```python
from build123d import *

# Parameters (mm, degrees)
SKETCH1_R               = 16.7005
SKETCH1_R_2             = 13.335
BOSS_EXTRUDE1_DEPTH     = 520.7
SKETCH3_R               = 16.7005
SKETCH3_R_2             = 13.335
BOSS_EXTRUDE2_DEPTH     = 660.4
SKETCH2_R               = 6.35
CUT_EXTRUDE1_DEPTH      = 17.7005
CUT_EXTRUDE1_DEPTH_BACK = 17.7005


with BuildPart() as part:
    # Sketch1 → Boss-Extrude1 (new body)
    with BuildSketch(Plane(origin=(0, 0, 0), x_dir=(1, 0, 0), z_dir=(0, 1, 0))):
        Circle(SKETCH1_R)
        Circle(SKETCH1_R_2, mode=Mode.SUBTRACT)
    extrude(amount=BOSS_EXTRUDE1_DEPTH)

    # Sketch3 → Boss-Extrude2 (add)
    with BuildSketch(Plane.XZ):
        Circle(SKETCH3_R)
        Circle(SKETCH3_R_2, mode=Mode.SUBTRACT)
    extrude(amount=BOSS_EXTRUDE2_DEPTH)

    # Sketch2 → Cut-Extrude1 (cut, two sides)
    with BuildSketch(Plane(origin=(0, 0, 0), x_dir=(0, 0, -1), z_dir=(1, 0, 0))) as cut_extrude1_sk:
        with Locations((0, -69.85)):
            Circle(SKETCH2_R)
    extrude(amount=CUT_EXTRUDE1_DEPTH, mode=Mode.SUBTRACT)
    extrude(cut_extrude1_sk.sketch, amount=-CUT_EXTRUDE1_DEPTH_BACK, mode=Mode.SUBTRACT)


solid = part.part
```
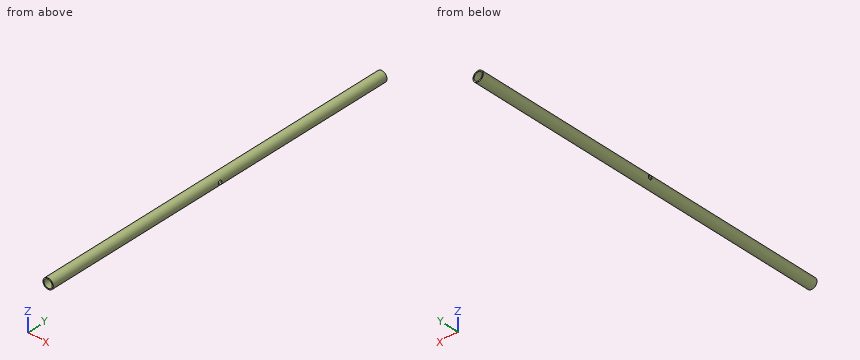
Part model, mm, in its own coordinate system. Coordinates: 2 decimals unless noted, no trailing zeros. Order: outer loops, then holes, each group sorted by start corner. A loop starts at its lowest first (then second) coordinate and runs counter-clockwise, first axis right, second up. Notation, with made-up numbers: (-6.5, -39) -> (50.5, -39) arc R16 cw to (50.5, -29) -> close; hole circle Ø9 at (-19, 31.5). An arc over 180 degrees is marked (long way). Put each result on its own line as item: value. Start each with the question number.
(1) Pin check, flat tips, straight feed: pin 1 Ø1 at (y, z) = (-254, 9) entering from +X; pin 2 Ø2 at (x, y) = (-7.5, 79) entering from +Z; pin 3 Ø4 at (x, y) = (3.5, -176.5) entering from +Z. Stop position of each tip, or through.
(2) Probe line 1 along X through (y, z) = (134.5, 1); line 2 along Z through (x, y) = (0, -124) (1 decimal); line 3 along X through (y, z) = (-53, -2). List the from-to ranges inside material, lowest first. Write a range as [from, to].
(3) Band-saw the part on C-C (y = 378). Give the cut face in (x, z) (1 decimal).
(4) Band-saw the part on A-A (x = 0). Give the cut face in (y, z) (1 decimal), then the cut area to 3 significant figures.
(5) Band-saw the part on B-B (z = 0). Give the cut face in (x, y) (1 decimal), then the cut area to 3 significant figures.
Determined:
1. pin 1: stops at x = 14.38
1. pin 2: stops at z = 15.38
1. pin 3: stops at z = 16.63
2. line 1: x = [-16.67, -13.3], [13.3, 16.67]
2. line 2: z = [-16.7, -13.3], [13.3, 16.7]
2. line 3: x = [-16.58, -13.18], [13.18, 16.58]
3. outline: circle Ø33.4 at (0, 0); hole circle Ø26.7 at (0, 0)
4. outline: (-660.4, -16.7) -> (520.7, -16.7) -> (520.7, -13.3) -> (-660.4, -13.3) -> close; (-660.4, 13.3) -> (520.7, 13.3) -> (520.7, 16.7) -> (-660.4, 16.7) -> close
4. area: 7,950 mm²
5. outline: (-16.7, -660.4) -> (-13.3, -660.4) -> (-13.3, -76.2) -> (-16.7, -76.2) -> close; (-16.7, -63.5) -> (-13.3, -63.5) -> (-13.3, 520.7) -> (-16.7, 520.7) -> close; (13.3, -660.4) -> (16.7, -660.4) -> (16.7, -76.2) -> (13.3, -76.2) -> close; (13.3, -63.5) -> (16.7, -63.5) -> (16.7, 520.7) -> (13.3, 520.7) -> close
5. area: 7,860 mm²
